Input: dimensioned drawing with shaded views. Units: mm. Origin: part minimum x, y, z. A direction names the side the tool comes from. Coordinates: 2 decimals unless noted, no trailing zeros. Loops run counter-clockwise (first coordinate to the right, second up) from the corner with the lowest first, then second, coordinate; pieces in that order, holes last. Notation, with made-up numbers: (5.5, 43.25) -> (51.5, 43.25) arc R27 cw to (51.5, 63.25) -> close; hole circle Ø10 at (79, 26). An arc over 180 degrees is marked (long way). Answer as CSV lines item,"result".
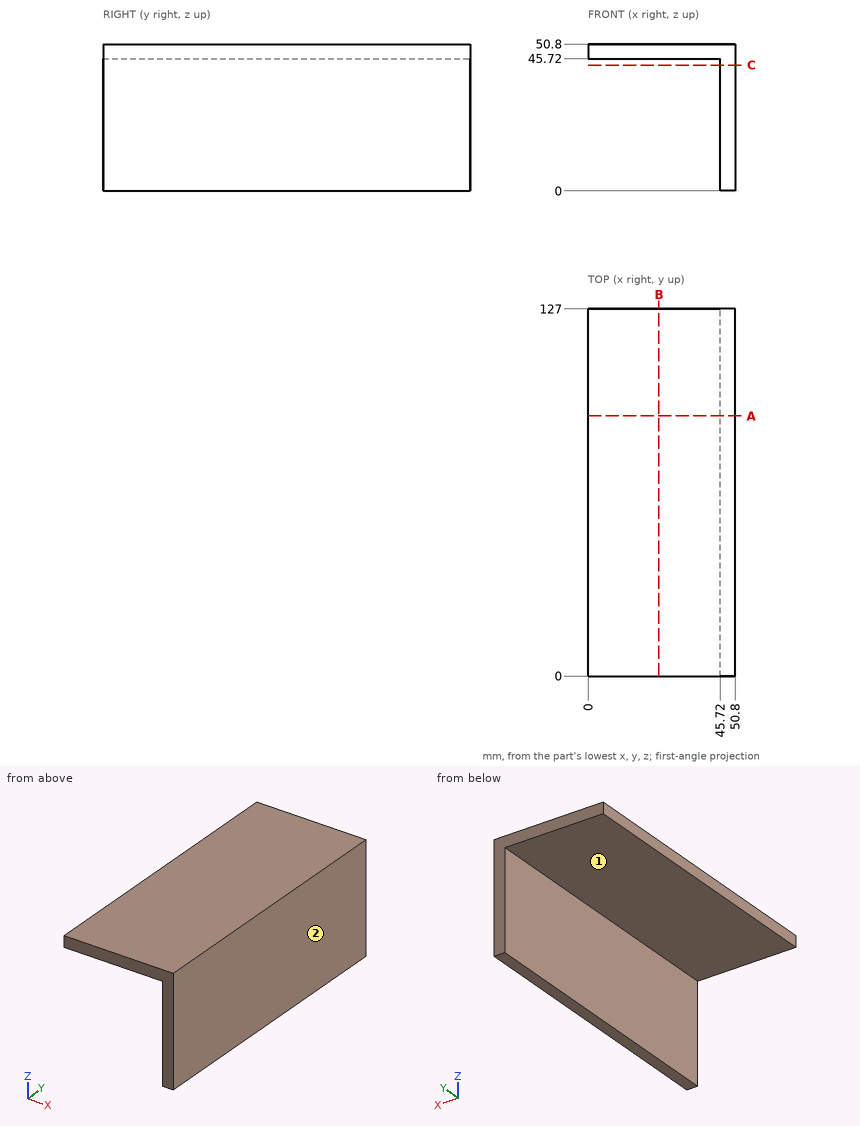
(1) Cut plane B-B (x = 24.5). Return the cut outline in (y, z).
Computed values:
outline,"(0, 45.72) -> (127, 45.72) -> (127, 50.8) -> (0, 50.8) -> close"
(2) Pin query (flat end, axial travel): pin 1 Ø23 at (y, z) = (68, 26.5) entering from -X; pin 2 Ø3 at (x, y) = (21, 83.5) entering from -Z. Return the tip coordinate at first contact, or that it passes through.
Computed values:
pin 1,"x = 45.72"
pin 2,"z = 45.72"
(3) Cut plane A-A (y = 90). Return the cut outline in (x, z), then the cut area to 3 significant figures.
Computed values:
outline,"(0, 45.72) -> (45.72, 45.72) -> (45.72, 0) -> (50.8, 0) -> (50.8, 50.8) -> (0, 50.8) -> close"
area,"490 mm^2"
(4) Access query for the marked faces 1 and 2. Directions: +Z, -Z, +X, -X, +Y, -Y. A direction counts if a zero-diameter tool reaches every point of the face in a straight line with its end or side. Return the directions, or none.
Computed values:
face 1,"-Z, -X, +Y, -Y"
face 2,"+Z, -Z, +X, +Y, -Y"
(5) Material intervals for L1, parallel to X at y = 26, z = 26.5, sorted ascending. Write a range as [from, to].
Computed values:
L1,"[45.72, 50.8]"
(6) Cut plane C-C (z = 43.5). Return the cut outline in (x, y), then the cut area to 3 significant figures.
Computed values:
outline,"(45.72, 0) -> (50.8, 0) -> (50.8, 127) -> (45.72, 127) -> close"
area,"645 mm^2"
